from build123d import *

# Parameters (mm, degrees)
SKETCH2_W           = 203.2
SKETCH2_H           = 12.7
SKETCH2_R           = 2.54
BOSS_EXTRUDE2_DEPTH = 2


with BuildPart() as part:
    # Sketch2 → Boss-Extrude2 (new, symmetric)
    with BuildSketch(Plane.XY):
        with Locations((0, 6.35)):
            Rectangle(SKETCH2_W, SKETCH2_H)
        with Locations((-96.562042846, 8.398896076)):
            Circle(SKETCH2_R, mode=Mode.SUBTRACT)
        with Locations((-50.984733006, 8.398896076)):
            Circle(SKETCH2_R, mode=Mode.SUBTRACT)
        with Locations(Location((96.562042846, 8.398896076, 0), (0, 0, 180))):
            Circle(SKETCH2_R, mode=Mode.SUBTRACT)
        with Locations((0, 8.398896076)):
            Circle(SKETCH2_R, mode=Mode.SUBTRACT)
        with Locations((50.984733006, 8.398896076)):
            Circle(SKETCH2_R, mode=Mode.SUBTRACT)
    extrude(amount=BOSS_EXTRUDE2_DEPTH, both=True)


solid = part.part
Geometry: final body of the model. Coordinates: model frame, mm. Round coordinates to 2 decimals unless told otherwise and drop trailing zeros. Order: outer loops, then holes, each group sorted by start corner. A loop starts at its lowest first (then second) coordinate and runs counter-clockwise, first axis right, second up. Notation, with made-up numbers: (-15.75, 27) - (-2.75, 27) arc R21 ccw to (-2.75, 63) - close; hole circle Ø1 at (56.5, 16). An arc over 180 degrees is marked (long way). Write each question's results on one line, items separated by ' | '.
Item 1: Section A-A, the plane x = 0. Return the cut outline in (y, z).
Completed:
outline: (0, -2) - (5.86, -2) - (5.86, 2) - (0, 2) - close; (10.94, -2) - (12.7, -2) - (12.7, 2) - (10.94, 2) - close
Item 2: First-contact query: pin 1 Ø4.5 at (x, y) = (50.98, 8.4) entering from +Z. Flat tip, straight axial feed; report the tip coordinate or a pass-through.
Completed:
pin 1: through
Item 3: Section B-B, the plane z = -1. Return the cut outline in (x, y), and give its area (3 significant figures).
Completed:
outline: (-101.6, 0) - (101.6, 0) - (101.6, 12.7) - (-101.6, 12.7) - close; hole circle Ø5.08 at (-96.56, 8.4); hole circle Ø5.08 at (-50.98, 8.4); hole circle Ø5.08 at (0, 8.4); hole circle Ø5.08 at (50.98, 8.4); hole circle Ø5.08 at (96.56, 8.4) | area: 2,480 mm^2
Item 4: Mould query, pull axis Y, two halves, no side actions, for faces 1 (the flat face through (-1, 0, 0)), 2 (the flat face through (101.6, 6, 0)), 3 (the cylindrical face through (-94.216, 7.426, -0.028)), 4 (the cylindrical face through (-0.55, 5.92, -0.03)). Classes: pulls with the +Y half, pulls with the -Y half, needs draft (parallel to the pull), parting line crosses it, or undercut.
Completed:
face 1: pulls with the -Y half | face 2: needs draft | face 3: undercut | face 4: undercut
Item 5: Material intervals for line 1 along X through (y, z) = (8.75, 1.65); line 2 along Y through (x, z) = (0, -0.65); line 3 along X through (y, z) = (7.25, 1.75), sorted ascending. Write a range as [from, to].
Completed:
line 1: [-101.6, -99.08], [-94.05, -53.5], [-48.47, -2.52], [2.52, 48.47], [53.5, 94.05], [99.08, 101.6] | line 2: [0, 5.86], [10.94, 12.7] | line 3: [-101.6, -98.83], [-94.3, -53.25], [-48.72, -2.27], [2.27, 48.72], [53.25, 94.3], [98.83, 101.6]
